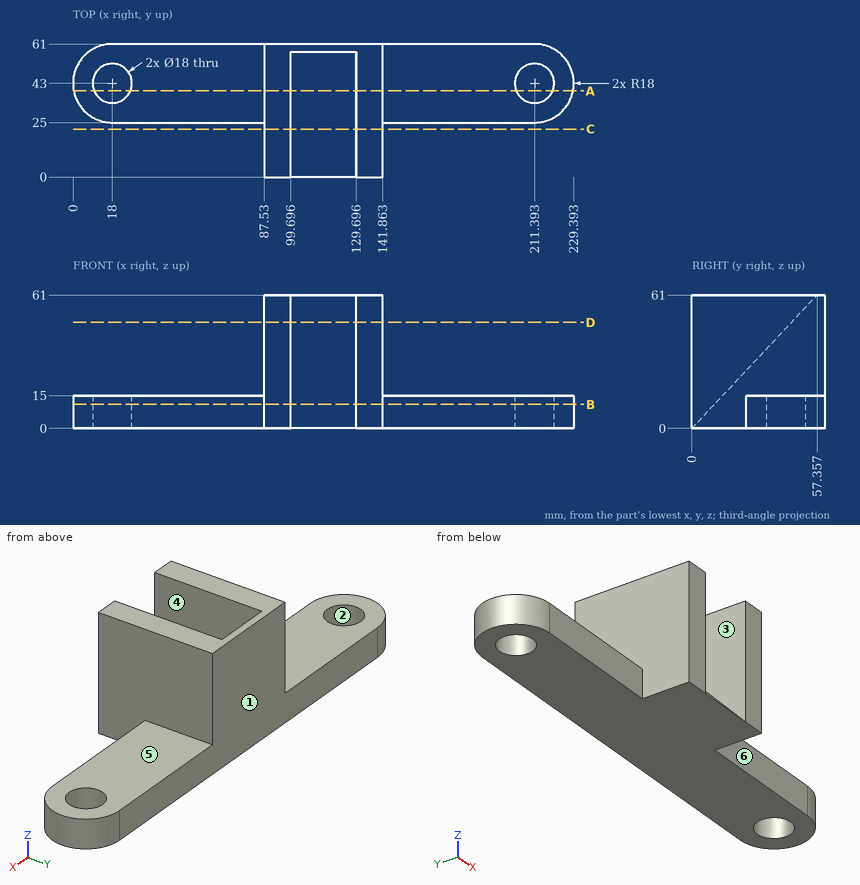
Design review of the part shown in the three views and the two pictorial views. Dimensions are in mm from the part's minimum x, y and z. A direction names the side the tool comes from. Give positions to 0.01 mm unless a question says otherwise; leave off trailing zeros. Loops run counter-clockwise (first coordinate to the right, second up) from the corner with the lowest first, then second, coordinate; pieces in that order, holes last. Notation, with made-up numbers: M 17,-16.75 L 66,-16.75 A36 ccw 66,19.25 Z; hole C 8.25,1 d9. An arc over 180 degrees is marked long. Answer as a JSON object with one key per item and string values. Group by question number.
Q1. Add section D-D on z = 48.5. Give the boundary of the cut face in (x, y).
Q2. For probe 1 along X at (y, z) = (15.5, 44); probe 2 along Y at (x, z) = (18, 11); probe 3 along X at (y, z) = (26, 20.5), list the stretches that pass through material, from the lowest coordinate up. Write a range as [from, to].
Q3. Add section B-B on z = 11. Give the boundary of the cut face in (x, y).
Q4. Add section A-A on y = 39.5. Give the number of separate pieces and of enclosed holes in the cut face, and give its area (3 significant figures).
Q5. Tool access review of the marked faces 4, 5 and 6: name each direction out of +Z, -Z, +X, -X, +Y, -Y from which nothing blocks a thin tool from reaching the whole face with its end or side.
Q6. Insertion check: P1, Ø10, axis at x = 58, y = 28, coming from the +Z side; P2, Ø16.5, axis at x = 48, z = 4, coming from the -Y side; P3, Ø1, axis at y = 54.5, z = 53.5, coming from the -X side. Each pin has a flat end and moves straight along its axis. Give the tip position at first contact, or say it passes through.
Q7. Add section C-C on y = 22. Give the boundary of the cut face in (x, z), and give its area (3 significant figures).
Q8. Mouldability with a two-part tool opening along Y and no side actions: class the marked faces 1, 2 and 3 as +Y half, -Y half, draft (parallel to the pull), parting line (faces both ways), or undercut.
Checked values:
{
 "1": {"outline": "M 87.53,0 L 99.7,0 L 99.7,45.6 L 129.7,45.6 L 129.7,0 L 141.86,0 L 141.86,61 L 87.53,61 Z"},
 "2": {"probe 1": "[87.53, 99.7], [129.7, 141.86]", "probe 2": "[25, 34], [52, 61]", "probe 3": "[87.53, 141.86]"},
 "3": {"outline": "M 18,25 L 87.53,25 L 87.53,0 L 99.7,0 L 99.7,10.34 L 129.7,10.34 L 129.7,0 L 141.86,0 L 141.86,25 L 211.39,25 A18 ccw 211.39,61 L 18,61 A18 ccw Z; hole C 18,43 d18; hole C 211.39,43 d18"},
 "4": {"separate pieces": "3", "enclosed holes": "0", "area": "4,860 mm²"},
 "5": {"face 4": "+Z, -Y", "face 5": "+Z, +X, +Y, -Y", "face 6": "+Z, -Z, +X, -Y"},
 "6": {"P1": "z = 15", "P2": "y = 25", "P3": "x = 87.53"},
 "7": {"outline": "M 87.53,0 L 141.86,0 L 141.86,61 L 129.7,61 L 129.7,23.4 L 99.7,23.4 L 99.7,61 L 87.53,61 Z", "area": "2,190 mm²"},
 "8": {"face 1": "+Y half", "face 2": "undercut", "face 3": "draft"}
}
